Part model, mm, in its own coordinate system. Face numbers are marked on the shaded views. A direction names the side the tool comes from. Give positions to 0.01 mm unless a question says otherwise; leave off trailing zeros. Write each loop counter-clockwise with the first axis right and the second up, starting at its lowest first coordinate (ties: lowest second). Pieces come first, ordered by that corner, then holes. Notation, with made-up numbers: M 25.25,38.5 L 35.25,38.5 A22 cw 35.25,57.5 Z; hole C 63.25,56.25 d2. An arc over 180 degrees is marked long. Write item = value, one per line. Start each with the question number.
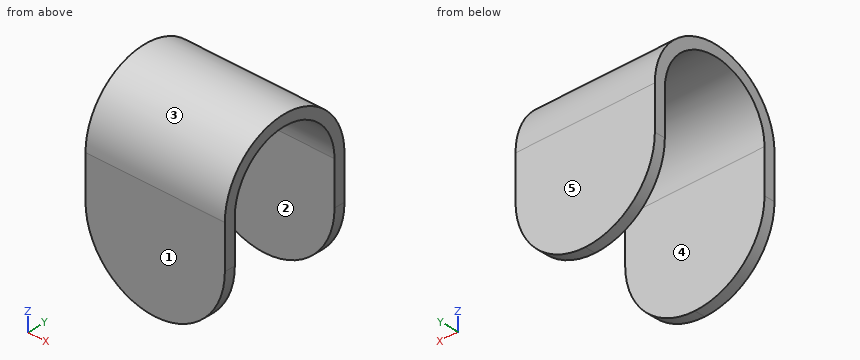
from build123d import *

# Parameters (mm, degrees)
F1_DEPTH = 41.275
F2_R     = 41.27499


# Not quite as in the source:
# - a fillet or chamfer is up to 0.001 mm smaller than in the source, because OpenCascade refuses the exact size


with BuildPart() as f1:
    # F0 (on Right) → F1 (new body, symmetric)
    with BuildSketch(Plane.YZ):
        with BuildLine():
            ThreePointArc((38.1, 0), (0, 38.1), (-38.1, 0))
            Line((-38.1, 0), (-38.1, -66.675))
            Line((-38.1, -66.675), (-31.75, -66.675))
            Line((-31.75, -66.675), (-31.75, 0))
            ThreePointArc((-31.75, 0), (0, 31.75), (31.75, 0))
            Line((31.75, 0), (31.75, -66.675))
            Line((31.75, -66.675), (38.1, -66.675))
            Line((38.1, -66.675), (38.1, 0))
        make_face()
    extrude(amount=F1_DEPTH, both=True)

    # F2 (radius 41.275 in the source; OpenCascade refuses exactly that, so slightly less here)
    f2_edges = [f1.edges().sort_by_distance(p)[0] for p in [
        (-41.275, 34.925, -66.675),
        (-41.275, -34.925, -66.675),
        (41.275, -34.925, -66.675),
        (41.275, 34.925, -66.675),
    ]]
    fillet(f2_edges, radius=F2_R)


solid = f1.part
Q1. Drop flat-ended pins along their axis: P1, Ø2, axis at x = 24, y = -27.5, coming from the -Z side; P2, Ø5, axis at x = -26, y = -26.5, coming from the -Z side; P3, Ø8, axis at x = 23, y = 7.5, coming from the +Z side. Give the stop position or say it passes through.
Q2. Slice it at D-D (y = 0). Give the cut face in (x, z) (3 decimals).
Q3. Slice it at C-C (z = -39). Give the cut face in (x, y).
Q4. Probe line 1 along Y through (x, z) = (-24, -51); line 2 along Y through (x, z) = (0, 11); line 3 along Z through (x, y) = (-25.5, 29). List the from-to ranges inside material, lowest first.
Q5. Slice it at A-A (z = -19.5). Give the cut face in (x, y) (3 decimals).
Q6. Tool access for the marked faces 1 and 2: list every direction of +Z, -Z, +X, -X, +Y, -Y with a clear straight run to the whole face (end or side of a thin tool).
Q7. Two-plate mould, pull along Y, no slides. Class the marked faces 3, 4 and 5: +Y half, -Y half, draft (parallel to the pull), parting line (faces both ways), or undercut.
Q8. Slice it at B-B (x = -28.5). Give the cut face in (y, z), and give its area (3 significant figures).
Working result:
q1.P1 = 13.99
q1.P2 = 12.93
q1.P3 = 37.94
q2.outline = M -41.275,31.75 L 41.275,31.75 L 41.275,38.1 L -41.275,38.1 Z
q3.outline = M -38.97,-38.1 L 38.97,-38.1 L 38.97,-31.75 L -38.97,-31.75 Z; M -38.97,31.75 L 38.97,31.75 L 38.97,38.1 L -38.97,38.1 Z
q4.line_1 = -38.1 to -31.75, 31.75 to 38.1
q4.line_2 = -36.48 to -29.78, 29.78 to 36.48
q4.line_3 = 12.93 to 24.71
q5.outline = M -41.275,-38.1 L 41.275,-38.1 L 41.275,-31.75 L -41.275,-31.75 Z; M -41.275,31.75 L 41.275,31.75 L 41.275,38.1 L -41.275,38.1 Z
q6.face_1 = +Z, -Z, +X, -X, -Y
q6.face_2 = -Z, +X, -X
q7.face_3 = parting line
q7.face_4 = undercut
q7.face_5 = +Y half
q8.outline = M -38.1,-55.26 L -31.75,-55.26 L -31.75,0 A31.75 cw 31.75,0 L 31.75,-55.26 L 38.1,-55.26 L 38.1,0 A38.1 ccw -38.1,0 Z
q8.area = 1,400 mm2
